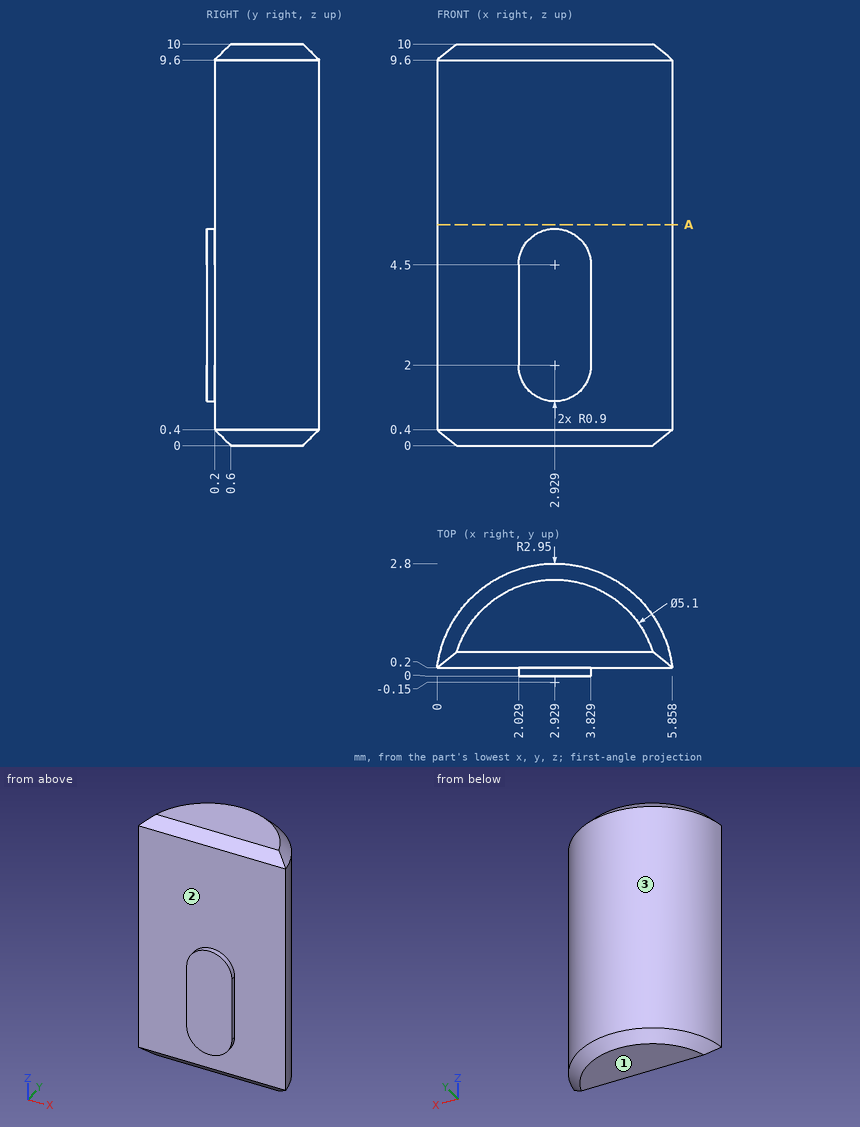
Job drawing, mm, ordinate dimensions from the low corner. One solid piece. Give positions to 0.01 mm unless a question says otherwise; leave off trailing zeros. Write each loop counter-clockwise with the first axis right and the second up, starting at its lowest first coordinate (ties: lowest second). Pieces come first, ordered by that corner, then holes. Notation, with made-up numbers: (-21.5, -4) -> (31.5, -4) arc R32 ccw to (31.5, 32) -> close; hole circle Ø8 at (71.25, -33.75). An arc over 180 degrees is marked (long way). Return JSON: item names as keys, results as strings.
Item 1: Drill centre lines: probe 1 along Z at (x, y) = (1.7, 0.55); probe 2 along Z at (x, y) = (1.5, 2.2); probe 3 along X at (y, z) = (1.95, 9.75) (1 decimal). Where is each one in solid material? Low to high.
Answer below:
{"probe 1": "z = 0.05 to 9.95", "probe 2": "z = 0.2 to 9.8", "probe 3": "x = 1.1 to 4.8"}
Item 2: Two-plate mould, pull along Y, no slides. Class the marked faces 1, 2 and 3: +Y half, -Y half, draft (parallel to the pull), parting line (faces both ways), or undercut.
Answer below:
{"face 1": "draft", "face 2": "-Y half", "face 3": "+Y half"}
Item 3: Drop flat-ended pins along their axis: pin 1 (1 mm diameter, centred on x = 0.5, z = 2.5, fed in from +Y); pin 2 (1 mm diameter, centred on x = 2, z = 2, fed in from -Y). Give the stop position or say it passes through.
Answer below:
{"pin 1": "stops at y = 2.08", "pin 2": "stops at y = 0"}
Item 4: Band-saw the part on A-A (z = 5.5). List the corners of the cut face in (x, y), then the cut area to 3 significant figures.
Answer below:
{"outline": "(0, 0.2) -> (5.86, 0.2) arc R2.95 ccw to start", "area": "11.6 mm2"}
